```python
from build123d import *

# Parameters (mm, degrees)
F0_R     = 10
F1_DEPTH = 10
F2_W     = 45
F2_H     = 8
F3_DEPTH = 20
F4_SIZE  = 5
F5_R     = 2
F6_T     = -1.5


with BuildPart() as f1:
    # F0 (on Front) → F1 (new body)
    with BuildSketch(Plane.XZ):
        with BuildLine():
            Line((-17.1517986995, 17.8985519321), (-17.1517986995, 5))
            ThreePointArc((-17.1517986995, 5), (-15.6873326054, 1.4644660941), (-12.1517986995, 0))
            Line((-12.1517986995, 0), (31.0146413554, 0))
            ThreePointArc((31.0146413554, 0), (35.0779397644, 2.0863071474), (35.7503227684, 6.6041575842))
            Line((35.7503227684, 6.6041575842), (26.0925432946, 35.115176199))
            ThreePointArc((26.0925432946, 35.115176199), (23.3227556246, 38.1083288927), (19.245201431, 38.0432244951))
            Line((19.245201431, 38.0432244951), (-14.2634591502, 22.4307578124))
            ThreePointArc((-14.2634591502, 22.4307578124), (-16.368331769, 20.585715655), (-17.1517986995, 17.8985519321))
        make_face()
        with Locations((12.0080858469, 14.3155753613)):
            Circle(F0_R, mode=Mode.SUBTRACT)
    extrude(amount=F1_DEPTH)

    # F2 (on Front) → F3 (join)
    with BuildSketch(Plane.XZ):
        with Locations((-25.4780513432, 4)):
            Rectangle(F2_W, F2_H)
    extrude(amount=F3_DEPTH)

    # F4
    f4_edges = [f1.edges().sort_by_distance(p)[0] for p in [
        (-2.978051, -20, 4),
    ]]
    chamfer(f4_edges, length=F4_SIZE)

    # F5
    f5_edges = [f1.edges().sort_by_distance(p)[0] for p in [
        (-17.151799, -10, 12.949276),
        (-16.368332, -10, 20.585716),
        (2.490871, -10, 30.236991),
        (23.322756, -10, 38.108329),
        (30.921433, -10, 20.859667),
        (35.07794, -10, 2.086307),
        (14.018295, -10, 0),
    ]]
    fillet(f5_edges, radius=F5_R)

    # F6
    f6_openings = [f1.faces().sort_by_distance(p)[0] for p in [
        (-47.978051, -10, 4),
    ]]
    offset(amount=F6_T, openings=f6_openings, kind=Kind.INTERSECTION)


solid = f1.part
```
Check sheet for the modelled part. Datum: model origin and axes. Units: mm. A direction names the side the tool comes from. Coordinates: 2 decimals unless noted, no trailing zeros. Order: outer loops, then holes, each group sorted by start corner. A loop starts at its lowest first (then second) coordinate and runs counter-clockwise, first axis right, second up. Notation, with made-up numbers: M -9,17 L 30,17 A26 cw 30,42 Z; hole C -24,8 d10. An arc over 180 degrees is marked long. One line per question, with ' | ' between items. Start each with the question number.
Item 1: Sectioned sample at B-B on x = 21. Count the separate pieces of the cut face and the enclosed holes in it, and give its area (3 significant figures).
Item 2: Sectioned sample at D-D on y = -17. Record the cut outline in (x, z).
Item 3: Mould release check, pull along Z, two halves, no side actions. Record for faces 4 (the cylindrical face through (23.377, -3.944, 38.085)), 5 (the flat face through (4, -8.5, 23)), 6 (the flat face through (3, 0, 20)): pulls with the +Z half, pulls with the -Z half, needs draft (parallel to the pull), parting line crosses it, or undercut.
Item 4: Sectioned sample at C-C on y = -13.5. Record the cut outline in (x, z), and give its area (4 significant figures).
Item 5: Material ranges on line 1 (Z direction, x = -31, y = -14); line 2 (Y direction, x = 14.5, z = 27); line 3 (X direction, y = -1.75, z = 10), recorded low to high.
Item 6: Gauge pin test, flat ends, axial feed: P1, Ø12, axis at x = 12.01, z = 14.32, coming from the -Y side; P2, Ø4, axis at y = -5, z = 15, coming from the +X side; P3, Ø1, axis at x = -16, y = -18, coming from the +Z side; P4, Ø5, axis at x = -10.5, y = -7, coming from the +Z side. Record the tip position at first contact, or that the pin passes through.
Item 7: Sectioned sample at A-A on y = -3.25. Record the cut outline in (x, z).
Item 8: Access from +Z, -Z, +X, -X, +Y, -Y to the whole of each face (thin tool, end or side, straight path). Record for faces 1 (the cylindrical face through (-16.55, -9.43, 12.88)), 2 (the flat face through (3.359, -4.704, 28.987)), 3 (the flat face through (-27, -10, 6.5)).
Answer below:
1) separate pieces: 2 | enclosed holes: 2 | area: 148 mm^2
2) outline: M -47.98,0 L -4.98,0 L -4.98,8 L -47.98,8 L -47.98,6.5 L -7.1,6.5 L -7.1,1.5 L -47.98,1.5 Z
3) face 4: pulls with the +Z half | face 5: undercut | face 6: needs draft
4) outline: M -47.98,0 L -2.98,0 L -2.98,8 L -47.98,8 L -47.98,6.5 L -4.48,6.5 L -4.48,1.5 L -47.98,1.5 Z | area: 142.5 mm^2
5) line 1: z = 0 to 1.5, 6.5 to 8 | line 2: y = -10 to -8.5, -1.5 to 0 | line 3: x = -17.15 to -15.65, 1.35 to 2.99, 21.03 to 22.67, 33.02 to 34.6
6) P1: passes through | P2: stops at x = 33.58 | P3: stops at z = 8 | P4: stops at z = 25.35
7) outline: M -47.98,0 L 31.01,0 A5 ccw 35.75,6.6 L 26.09,35.12 A5 ccw 19.25,38.04 L -14.26,22.43 A5 ccw -17.15,17.9 L -17.15,8 L -47.98,8 L -47.98,6.5 L -15.65,6.5 L -15.65,17.9 A3.5 cw -13.63,21.07 L 19.88,36.68 A3.5 cw 24.67,34.63 L 34.33,6.12 A3.5 cw 31.01,1.5 L -47.98,1.5 Z; C 12.01,14.32 d23; hole C 12.01,14.32 d20
8) face 1: +Z, -X, -Y | face 2: none | face 3: -X
